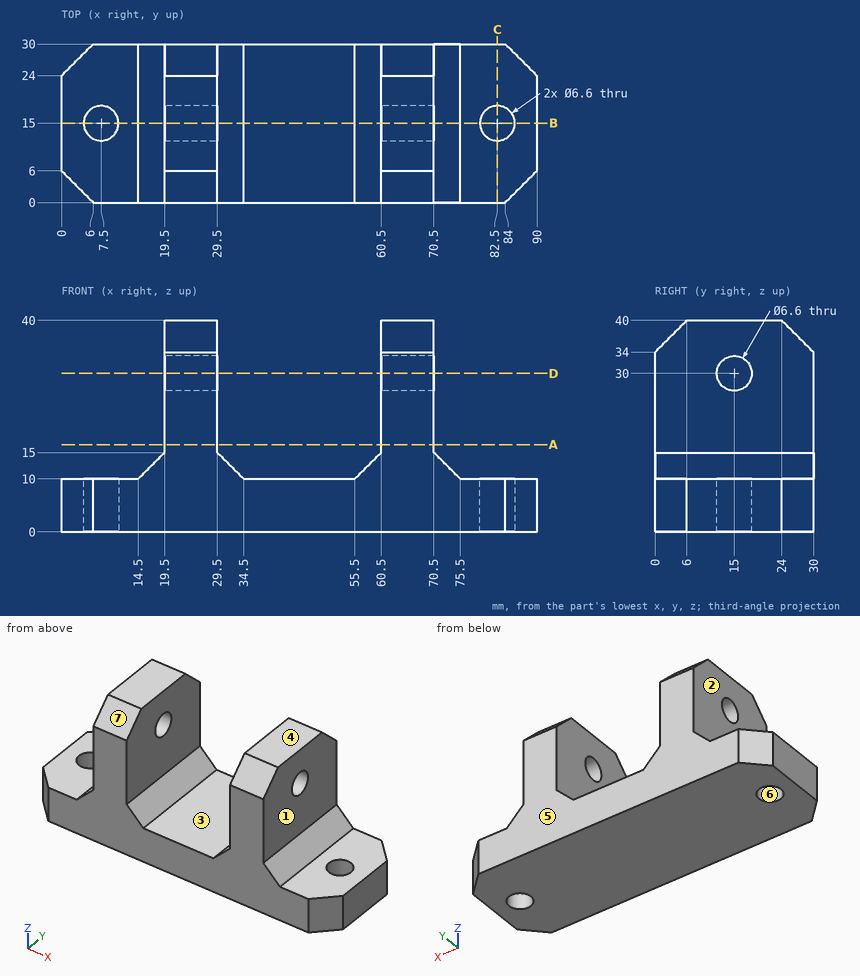
Input: dimensioned drawing with shaded views. Units: mm. Origin: part minimum x, y, z. A direction names the side the tool comes from. Round coordinates to 2 decimals unless told otherwise and drop trailing zeros. Loops run counter-clockwise (first coordinate to the right, second up) from the corner with the lowest first, then second, coordinate; pieces in that order, holes last. Notation, with made-up numbers: (73, 50) -> (129, 50) arc R22 cw to (129, 83) -> close; hole circle Ø9 at (-10, 16). An arc over 180 degrees is marked (long way). One line per item, written item: value.
(1) Pin query (flat end, axial travel): pin 1 (6.5 mm diameter, centred on x = 43.5, y = 17.5, fed in from +Z); pin 2 (1.5 mm diameter, centred on y = 15, z = 15, fed in from +X); pin 3 (12 mm diameter, centred on y = 15.5, z = 20.5, fed in from +X); pin 4 (6 mm diameter, centred on x = 7.5, y = 15, fed in from +Z). Return the tip coordinate at first contact, or that it passes through.
Geometry check:
pin 1: z = 10
pin 2: x = 71.25
pin 3: x = 71
pin 4: through
(2) Section C-C (x = 82.5). Return the cut outline in (y, z).
Geometry check:
outline: (0, 0) -> (11.7, 0) -> (11.7, 10) -> (0, 10) -> close; (18.3, 0) -> (30, 0) -> (30, 10) -> (18.3, 10) -> close
(3) Section D-D (z = 30). Return the cut outline in (x, y).
Geometry check:
outline: (19.5, 0) -> (29.5, 0) -> (29.5, 11.7) -> (19.5, 11.7) -> close; (19.5, 18.3) -> (29.5, 18.3) -> (29.5, 30) -> (19.5, 30) -> close; (60.5, 0) -> (70.5, 0) -> (70.5, 11.7) -> (60.5, 11.7) -> close; (60.5, 18.3) -> (70.5, 18.3) -> (70.5, 30) -> (60.5, 30) -> close
(4) Section B-B (y = 15). Give the number of separate pieces and of enclosed holes in the cut face, plus the area to 3 significant figures.
Geometry check:
separate pieces: 5
enclosed holes: 0
area: 1,290 mm2
(5) Mould query, pull axis Y, two halves, no side actions, for the marked faces 4, 5, 6 and 7. Classes: pulls with the +Y half, pulls with the -Y half, needs draft (parallel to the pull), parting line crosses it, or undercut.
Geometry check:
face 4: needs draft
face 5: pulls with the +Y half
face 6: undercut
face 7: pulls with the -Y half
(6) Section A-A (z = 16.5). Return the cut outline in (x, y).
Geometry check:
outline: (19.5, 0) -> (29.5, 0) -> (29.5, 30) -> (19.5, 30) -> close; (60.5, 0) -> (70.5, 0) -> (70.5, 30) -> (60.5, 30) -> close
(7) Material intervals for line 1 (Y direction, x = 7.5, z = 5.5); line 2 (X direction, y = 18.75, z = 36); line 3 (Z direction, x = 67.75, y = 15), sorted ascending. Write a range as [from, to].
Geometry check:
line 1: [0, 11.7], [18.3, 30]
line 2: [19.5, 29.5], [60.5, 70.5]
line 3: [0, 26.7], [33.3, 40]
(8) Set-up query: the marked faces 1, 2 and 3. Return all of +Z, -Z, +X, -X, +Y, -Y with unobstructed straight access to the full face (end or side cutting, diameter ignored); none if empty.
Geometry check:
face 1: +Z, +X, +Y, -Y
face 2: +Z, -X, +Y, -Y
face 3: +Z, +Y, -Y
